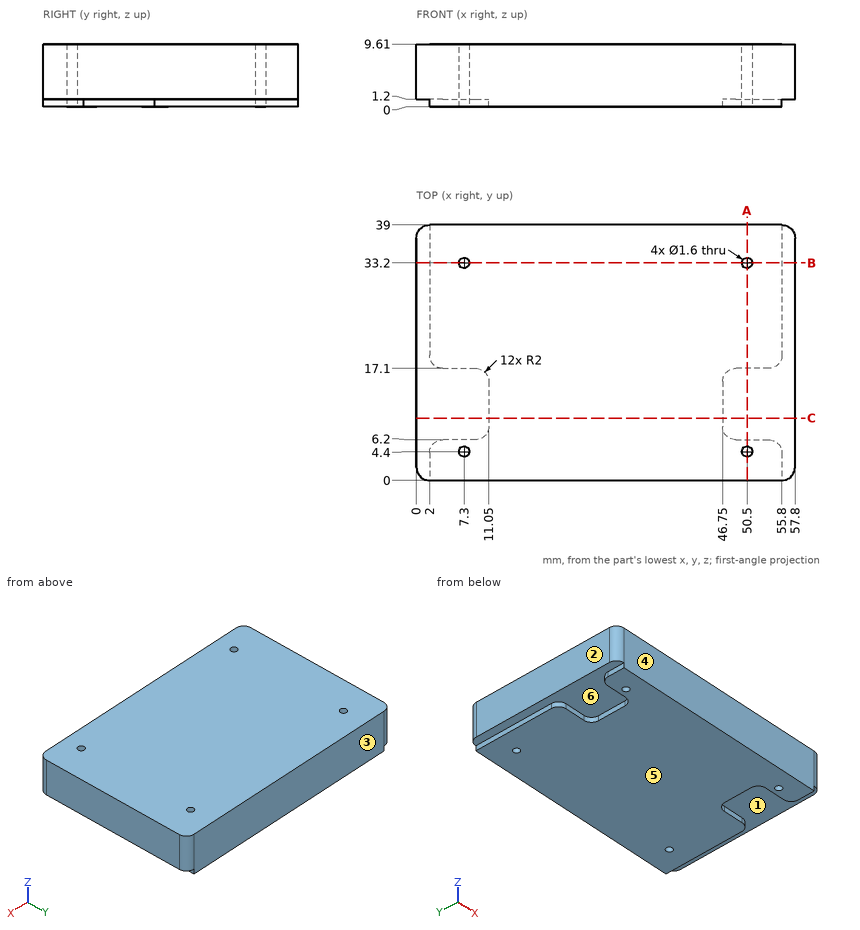
For this review, use the dimensioned drawing (mm, ordinates from the lowest corner) and the shaded views. A direction names the side the tool comes from. Give positions to 0.01 mm unless a question says otherwise; leave off trailing zeros. Order: outer loops, then holes, each group sorted by start corner. A loop starts at its lowest first (then second) coordinate and runs counter-clockwise, first axis right, second up.
1) For the marked faces 5 and 6, list the 3-axis set-ups (+Z, -Z, +X, -X, +Y, -Y) from which the entire face can be reached by the end or side of a thin tool; tool diameter is ignored.
2) Insertion check: pin 1 (0.6 mm diameter, centred on y = 11, z = 0.5, fed in from +X); pin 2 (1 mm diameter, centred on y = 2, z = 0.5, fed in from +X); pin 3 (0.6 mm diameter, centred on y = 12, z = 0.5, fed in from -X). Each pin has a flat end and moves straight along its axis. Give the tip position at first contact, or say it passes through.
3) Take a section at A-A (x = 50.5). Give the boundary of the cut face in (y, z).
4) The part is to be moulded in two halves that separate along Y. For the marked faces 1, 2, 3 and 4, say which applies: released by +Y, released by -Y, zero draft, split by the parting line, or undercut.
5) Take a section at C-C (y = 9.5). Give the boundary of the cut face in (x, z), then the cut area to 3 significant figures.
6) Take a section at B-B (y = 33.2). Give the boundary of the cut face in (x, z).
7) Wall thickness on line 1 (Y direction, x = 50.5, z = 4.25); line 2 (X direction, y = 4.5, z = 3); line 3 (Y direction, x = 51, z = 6.25): over which ranges is each line inside the solid? List them lowest first.
Derived:
1. face 5: -Z, +X, -X, +Y, -Y
1. face 6: -Z, -X
2. pin 1: stops at x = 46.75
2. pin 2: stops at x = 55.8
2. pin 3: stops at x = 11.05
3. outline: (0, 0) - (3.6, 0) - (3.6, 9.61) - (0, 9.61) - close; (5.2, 0) - (6.2, 0) - (6.2, 1.2) - (17.1, 1.2) - (17.1, 0) - (32.4, 0) - (32.4, 9.61) - (5.2, 9.61) - close; (34, 0) - (39, 0) - (39, 9.61) - (34, 9.61) - close
4. face 1: undercut
4. face 2: zero draft
4. face 3: released by +Y
4. face 4: released by -Y
5. outline: (0, 1.2) - (11.05, 1.2) - (11.05, 0) - (46.75, 0) - (46.75, 1.2) - (57.8, 1.2) - (57.8, 9.61) - (0, 9.61) - close
5. area: 529 mm2
6. outline: (0, 1.2) - (2, 1.2) - (2, 0) - (6.5, 0) - (6.5, 9.61) - (0, 9.61) - close; (8.1, 0) - (49.7, 0) - (49.7, 9.61) - (8.1, 9.61) - close; (51.3, 0) - (55.8, 0) - (55.8, 1.2) - (57.8, 1.2) - (57.8, 9.61) - (51.3, 9.61) - close
7. line 1: y = 0 to 3.6, 5.2 to 32.4, 34 to 39
7. line 2: x = 0 to 6.51, 8.09 to 49.71, 51.29 to 57.8
7. line 3: y = 0 to 3.78, 5.02 to 32.58, 33.82 to 39
